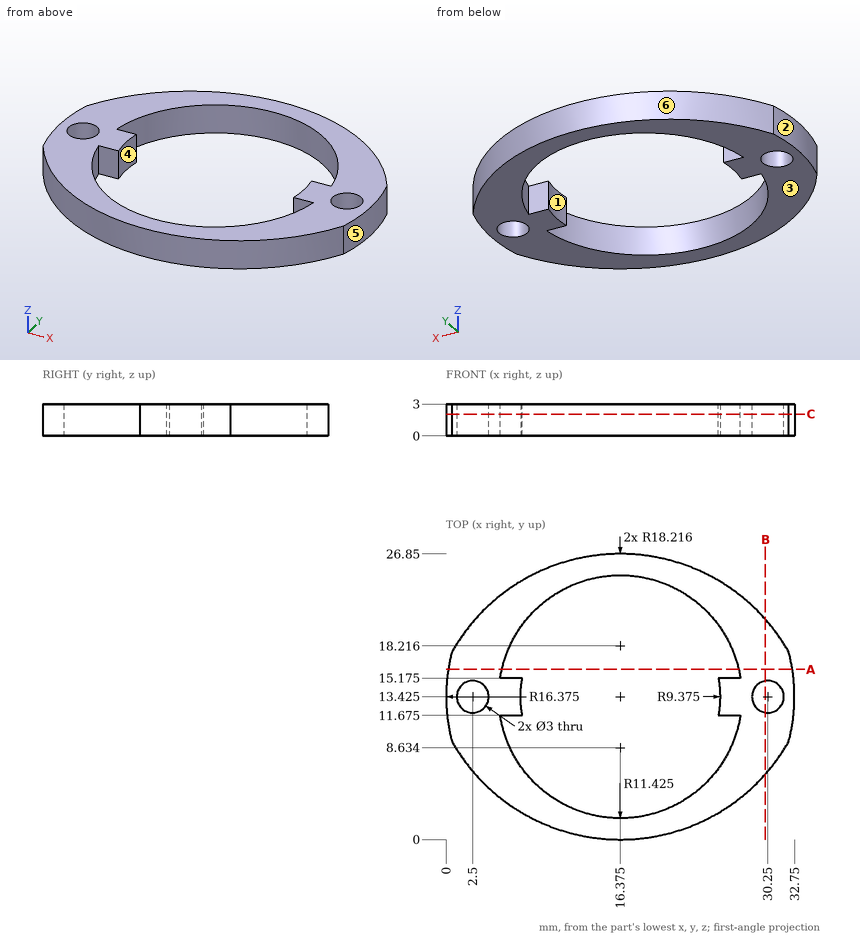
Could you check a few things on this drawing? It's one solid part, dimensions in mm from its lowest x, y, z. A direction names the side the tool comes from. Coordinates: 2 decimals unless noted, no trailing zeros. Write each loop counter-clockwise with the first axis right and the second up, starting at its lowest first coordinate (ties: lowest second). Pieces come first, ordered by that corner, then holes. Notation, with made-up numbers: (-20.75, 42.5) - (29.25, 42.5) arc R3 cw to (29.25, 47.5) - close; hole circle Ø8 at (10.25, -15). An arc over 180 degrees is marked (long way). Return JSON: item names as keys, results as strings. Group by question number.
Item 1: Which directions (+Z, -Z, +X, -X, +Y, -Y) give clear straight access to the entire face, cutting with the end or side of a thin tool? Please do the marked faces 1 and 2.
Item 2: We'd pull the mould along Y, two halves only. Please class the marked faces 3, 4, 5 and 6: pulls with the +Y half, pulls with the -Y half, needs draft (parallel to the pull), parting line crosses it, or undercut.
Item 3: If we section it at A-A (y = 16): Write out the boundary of the cut face in (x, z).
Item 4: Please list where these lines run through material, in increasing order: probe 1 along X at (y, z) = (12.25, 1.3) (1 decimal); probe 2 along Y at (x, z) = (26.5, 1.75) (1 decimal); probe 3 along Y at (x, z) = (30.25, 1.8) (1 decimal).
Item 5: If we section it at B-B (x = 30): Write out the boundary of the cut face in (y, z).
Item 6: I'm going to push flat-ended pins straight in: pin 1 Ø1.7 at (x, z) = (5.5, 1) entering from +Y; pin 2 Ø1.7 at (x, z) = (6, 2) entering from -Y; pin 3 Ø1.5 at (y, z) = (5.5, 0.5) entering from -X. Where does each tip first touch, or does it pass through?
Item 7: If we section it at C-C (z = 2.05): Count the separate pieces of the cut face and the enclosed holes in it, then the cut area to 3 significant figures.
Return value:
{
 "1": {"face 1": "+Z, -Z", "face 2": "+Z, -Z, -X"},
 "2": {"face 3": "needs draft", "face 4": "undercut", "face 5": "parting line crosses it", "face 6": "pulls with the +Y half"},
 "3": {"outline": "(0.2, 0) - (5.24, 0) - (5.24, 3) - (0.2, 3) - close; (27.51, 0) - (32.55, 0) - (32.55, 3) - (27.51, 3) - close"},
 "4": {"probe 1": "x = 0 to 1.6, 3.4 to 7.1, 25.7 to 29.3, 31.2 to 32.7", "probe 2": "y = 3.1 to 8.1, 11.7 to 15.2, 18.7 to 23.8", "probe 3": "y = 6.4 to 11.9, 14.9 to 20.4"},
 "5": {"outline": "(6.13, 0) - (11.95, 0) - (11.95, 3) - (6.13, 3) - close; (14.9, 0) - (20.72, 0) - (20.72, 3) - (14.9, 3) - close"},
 "6": {"pin 1": "stops at y = 23.84", "pin 2": "stops at y = 2.69", "pin 3": "stops at x = 2.64"},
 "7": {"separate pieces": "1", "enclosed holes": "3", "area": "277 mm^2"}
}
